Source: CAD feature listing. Evaluate the final solid. Frame: model axes, mm. Face numbers are marked on the shaded views. Give positions to 0.01 mm unless a question says otherwise; leave off trailing zeros. Write each loop counter-clockwise with the first axis right and the second up, starting at its lowest first coordinate (ties: lowest second). Pieces come first, ordered by that corner, then holes. Notation, with made-up numbers: (88.25, -14) -> (128.25, -14) arc R29 ccw to (128.25, 18) -> close; hole circle Ø6 at (4, 89.5). An arc over 180 degrees is marked (long way). Answer as a JSON object with one key per item and string values. Group by question number.
Item 1: Section query B-B on x = -8. Return the cut outline in (y, z), plus the area to 3 significant figures.
Item 2: Pull-direction query (Y, two-part tool) for the marked faces 1 and 2; classes: pulls with the +Y half, pulls with the -Y half, needs draft (parallel to the pull), parting line crosses it, or undercut.
Item 3: Section query A-A on y = 4. Return the cut outline in (x, z).
Item 4: Ray query, probe 1 along X at (y, z) = (10, 2); probe 2 along Y at (x, z) = (0, 1.35); probe 3 along Y at (x, z) = (8, 1.45). Return the intervals inside material, ascending. Write a range as from..to.
Item 5: Section query C-C on z = 0.6. Give the number of separate pieces and of enclosed holes in the cut face, plus the area to 3 significant figures.
Item 6: Section query D-D on y = -11. Return the cut outline in (x, z), plus the area to 3 significant figures.
from build123d import *

# Parameters (mm, degrees)
F0_W     = 42
F0_H     = 30
F1_DEPTH = 3
F2_D     = 3
F3_D     = 3.1
F4_D     = 3.2
F5_D     = 3.3
F6_D     = 3.4
F7_D     = 3.5
F8_D     = 3.6
F9_D     = 3.7
F10_D    = 3.8
F11_D    = 3.9
F12_D    = 4
F13_D    = 4.1
F14_D    = 4.2
F15_D    = 4.3
F16_D    = 4.4
F17_D    = 4.5
F18_D    = 4.6
F19_D    = 4.7
F20_D    = 4.8
F21_D    = 4.9


with BuildPart() as f1:
    # F0 (on Top) → F1 (new body)
    with BuildSketch(Plane.XY):
        Rectangle(F0_W, F0_H)
    extrude(amount=F1_DEPTH)

    # F2 (through all)
    with Locations(Plane(origin=(0, 0, 0), x_dir=(1, 0, 0), z_dir=(0, 0, -1))):
        with Locations((-16, -10)):
            Hole(F2_D / 2)

    # F3 (through all)
    with Locations(Plane(origin=(0, 0, 0), x_dir=(1, 0, 0), z_dir=(0, 0, -1))):
        with Locations((-8, -10)):
            Hole(F3_D / 2)

    # F4 (through all)
    with Locations(Plane(origin=(0, 0, 0), x_dir=(1, 0, 0), z_dir=(0, 0, -1))):
        with Locations((0, -10)):
            Hole(F4_D / 2)

    # F5 (through all)
    with Locations(Plane(origin=(0, 0, 0), x_dir=(1, 0, 0), z_dir=(0, 0, -1))):
        with Locations((8, -10)):
            Hole(F5_D / 2)

    # F6 (through all)
    with Locations(Plane(origin=(0, 0, 0), x_dir=(1, 0, 0), z_dir=(0, 0, -1))):
        with Locations((16, -10)):
            Hole(F6_D / 2)

    # F7 (through all)
    with Locations(Plane(origin=(0, 0, 0), x_dir=(1, 0, 0), z_dir=(0, 0, -1))):
        with Locations((-16, -4)):
            Hole(F7_D / 2)

    # F8 (through all)
    with Locations(Plane(origin=(0, 0, 0), x_dir=(1, 0, 0), z_dir=(0, 0, -1))):
        with Locations((-8, -4)):
            Hole(F8_D / 2)

    # F9 (through all)
    with Locations(Plane(origin=(0, 0, 0), x_dir=(1, 0, 0), z_dir=(0, 0, -1))):
        with Locations((0, -4)):
            Hole(F9_D / 2)

    # F10 (through all)
    with Locations(Plane(origin=(0, 0, 0), x_dir=(1, 0, 0), z_dir=(0, 0, -1))):
        with Locations((8, -4)):
            Hole(F10_D / 2)

    # F11 (through all)
    with Locations(Plane(origin=(0, 0, 0), x_dir=(1, 0, 0), z_dir=(0, 0, -1))):
        with Locations((16, -4)):
            Hole(F11_D / 2)

    # F12 (through all)
    with Locations(Plane(origin=(0, 0, 0), x_dir=(1, 0, 0), z_dir=(0, 0, -1))):
        with Locations((-16, 3)):
            Hole(F12_D / 2)

    # F13 (through all)
    with Locations(Plane(origin=(0, 0, 0), x_dir=(1, 0, 0), z_dir=(0, 0, -1))):
        with Locations((-8, 3)):
            Hole(F13_D / 2)

    # F14 (through all)
    with Locations(Plane(origin=(0, 0, 0), x_dir=(1, 0, 0), z_dir=(0, 0, -1))):
        with Locations((0, 3)):
            Hole(F14_D / 2)

    # F15 (through all)
    with Locations(Plane(origin=(0, 0, 0), x_dir=(1, 0, 0), z_dir=(0, 0, -1))):
        with Locations((8, 3)):
            Hole(F15_D / 2)

    # F16 (through all)
    with Locations(Plane(origin=(0, 0, 0), x_dir=(1, 0, 0), z_dir=(0, 0, -1))):
        with Locations((16, 3)):
            Hole(F16_D / 2)

    # F17 (through all)
    with Locations(Plane(origin=(0, 0, 0), x_dir=(1, 0, 0), z_dir=(0, 0, -1))):
        with Locations((-16, 11)):
            Hole(F17_D / 2)

    # F18 (through all)
    with Locations(Plane(origin=(0, 0, 0), x_dir=(1, 0, 0), z_dir=(0, 0, -1))):
        with Locations((-8, 11)):
            Hole(F18_D / 2)

    # F19 (through all)
    with Locations(Plane(origin=(0, 0, 0), x_dir=(1, 0, 0), z_dir=(0, 0, -1))):
        with Locations((0, 11)):
            Hole(F19_D / 2)

    # F20 (through all)
    with Locations(Plane(origin=(0, 0, 0), x_dir=(1, 0, 0), z_dir=(0, 0, -1))):
        with Locations((8, 11)):
            Hole(F20_D / 2)

    # F21 (through all)
    with Locations(Plane(origin=(0, 0, 0), x_dir=(1, 0, 0), z_dir=(0, 0, -1))):
        with Locations((16, 11)):
            Hole(F21_D / 2)


solid = f1.part
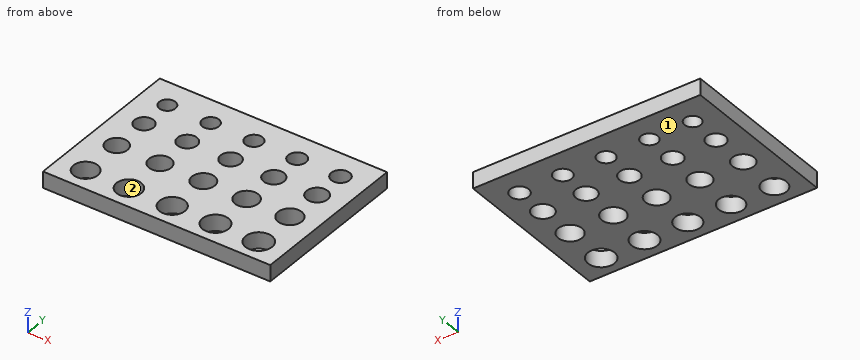
Worked answers:
{
 "1": {"outline": "(-15, 0) -> (-13.3, 0) -> (-13.3, 3) -> (-15, 3) -> close; (-8.7, 0) -> (-5.05, 0) -> (-5.05, 3) -> (-8.7, 3) -> close; (-0.95, 0) -> (2.2, 0) -> (2.2, 3) -> (-0.95, 3) -> close; (5.8, 0) -> (8.45, 0) -> (8.45, 3) -> (5.8, 3) -> close; (11.55, 0) -> (15, 0) -> (15, 3) -> (11.55, 3) -> close", "area": "43.8 mm^2"},
 "2": {"face 1": "needs draft", "face 2": "undercut"},
 "3": {"outline": "(-21, 0) -> (-17.75, 0) -> (-17.75, 3) -> (-21, 3) -> close; (-14.25, 0) -> (-9.8, 0) -> (-9.8, 3) -> (-14.25, 3) -> close; (-6.2, 0) -> (-1.85, 0) -> (-1.85, 3) -> (-6.2, 3) -> close; (1.85, 0) -> (6.1, 0) -> (6.1, 3) -> (1.85, 3) -> close; (9.9, 0) -> (14.05, 0) -> (14.05, 3) -> (9.9, 3) -> close; (17.95, 0) -> (21, 0) -> (21, 3) -> (17.95, 3) -> close"},
 "4": {"probe 1": "-21..-17.5, -14.5..-9.55, -6.45..-1.6, 1.6..6.35, 9.65..14.3, 17.7..21", "probe 2": "-15..-13.35, -8.65..-5.1, -0.9..2.15, 5.85..8.4, 11.6..15", "probe 3": "-15..-13.4, -8.6..-5.15, -0.85..2.1, 5.9..8.35, 11.65..15"},
 "5": {"separate pieces": "1", "enclosed holes": "20", "area": "1,010 mm^2"},
 "6": {"outline": "(-21, 0) -> (-18.25, 0) -> (-18.25, 3) -> (-21, 3) -> close; (-13.75, 0) -> (-10.3, 0) -> (-10.3, 3) -> (-13.75, 3) -> close; (-5.7, 0) -> (-2.35, 0) -> (-2.35, 3) -> (-5.7, 3) -> close; (2.35, 0) -> (5.6, 0) -> (5.6, 3) -> (2.35, 3) -> close; (10.4, 0) -> (13.55, 0) -> (13.55, 3) -> (10.4, 3) -> close; (18.45, 0) -> (21, 0) -> (21, 3) -> (18.45, 3) -> close", "area": "55.5 mm^2"}
}
